```python
from build123d import *

# Parameters (mm, degrees)
SKETCH2_W = 3
SKETCH2_H = 4


with BuildPart() as part:
    # Sweep1: sweep along a path in Sketch1
    with BuildLine(Plane(origin=(0, 0, 0), x_dir=(1, 0, 0), z_dir=(0, 1, 0))) as sweep1_path:
        Line((-1.391672956, 4.489236726), (71.138118239, 26.973626627))
        ThreePointArc((71.138118239, 26.973626627), (107.74, 0), (71.138118239, -26.973626627))
        Line((71.138118239, -26.973626627), (-1.391672956, -4.489236726))
        ThreePointArc((-1.391672956, -4.489236726), (-4.7, 0), (-1.391672956, 4.489236726))
    # Sketch2 → Sweep1 (sweep)
    with BuildSketch(Plane(origin=(79.5, 0, 0), x_dir=(0, 0, -1), z_dir=(1, 0, 0))):
        with Locations((29.74, 0)):
            Rectangle(SKETCH2_W, SKETCH2_H)
    sweep(path=sweep1_path.line)


solid = part.part
```
Work out the finished part from the listing and answer in its coordinate system (mm). A direction names the side the tool comes from. Give positions to 0.01 mm unless a question says otherwise; leave off trailing zeros. Write each loop counter-clockwise with the first axis right and the second up, starting at its lowest first coordinate (ties: lowest second). Pieces come first, ordered by that corner, then holes. Notation, with made-up numbers: (56, -25.5) - (110, -25.5) arc R23 cw to (110, -0.5) - close; hole circle Ø3 at (24, -6.75). An arc over 180 degrees is marked (long way). Use one line per item in the form item = value.
1. A cutting plane is placed at B-B (x = 95.5). Write down the section's boundary in (y, z).
Filled in:
outline = (-2, -26.83) - (2, -26.83) - (2, -23.27) - (-2, -23.27) - close; (-2, 23.27) - (2, 23.27) - (2, 26.83) - (-2, 26.83) - close
2. Consider L1, parallel to X at y = -0.65, z = 0; L2, parallel to Z at x = 79.5, y = -0.55; L3, parallel to Z at x = 41.5, y = -0.4. Determine where each line is inside the solid, lowest interval first.
Filled in:
L1 = -7.7 to -4.7, 107.74 to 110.74
L2 = -31.24 to -28.24, 28.24 to 31.24
L3 = -20.93 to -17.79, 17.79 to 20.93
3. This flat-tipped pin is pushed along its axis until it touches: pin 1 Ø1 at (y, z) = (0.5, 12.5) entering from +X. Where does it stop, or does it pass through?
Filled in:
pin_1 = 108.34
4. A cutting plane is placed at C-C (y = 0.55). Write down the section's boundary in (x, z).
Filled in:
outline = (-2.28, -7.35) - (70.25, -29.84) arc R31.24 ccw (long way) to (70.25, 29.84) - (-2.28, 7.35) arc R7.7 ccw to start; hole (-1.39, -4.49) - (71.14, -26.97) arc R28.24 ccw (long way) to (71.14, 26.97) - (-1.39, 4.49) arc R4.7 ccw to start
5. Determine the mould class of faces 1 (the face through (110.73, 0.03, -0.82)), 2 (the face through (54.8, -2, 22.3)), 3 (the face through (34.366, 0.028, 15.574)), 4 (the face through (-4.7, 0, 0.1)) for opening direction X: released by +X, released by -X, zero draft, split by the parting line, or undercut.
Filled in:
face_1 = split by the parting line
face_2 = zero draft
face_3 = undercut
face_4 = undercut
6. A cutting plane is placed at A-A (z = 0). Write down the section's boundary in (x, y), and give its area (3 significant figures).
Filled in:
outline = (-7.7, -2) - (-4.7, -2) - (-4.7, 2) - (-7.7, 2) - close; (107.74, -2) - (110.74, -2) - (110.74, 2) - (107.74, 2) - close
area = 24.0 mm^2
7. For faces 5 (the face through (35.38, 0.03, -15.89)), 6 (the face through (54.7, 2, 22.1)), determine the directions among +Z, -Z, +X, -X, +Y, -Y from which every point of the face is accessible in a straight line to the end or side of a thin tool.
Filled in:
face_5 = +Y, -Y
face_6 = +Z, -Z, +X, -X, +Y
